Verification items for this drawing (mm, ordinates from the low corner). A direction names the side the tool comes from. Give positions to 0.01 mm unless a question says otherwise; leave off trailing zeros. Loops run counter-clockwise (first coordinate to the right, second up) from the corner with the lowest first, then second, coordinate; pieces in that order, holes last. Notation, with made-up numbers: M 24,62 L 69,62 A22 ccw 69,70 Z; hole C 87.5,-25.75 d3. An arc over 180 degrees is marked long. Answer in a Markdown table with one row per item.
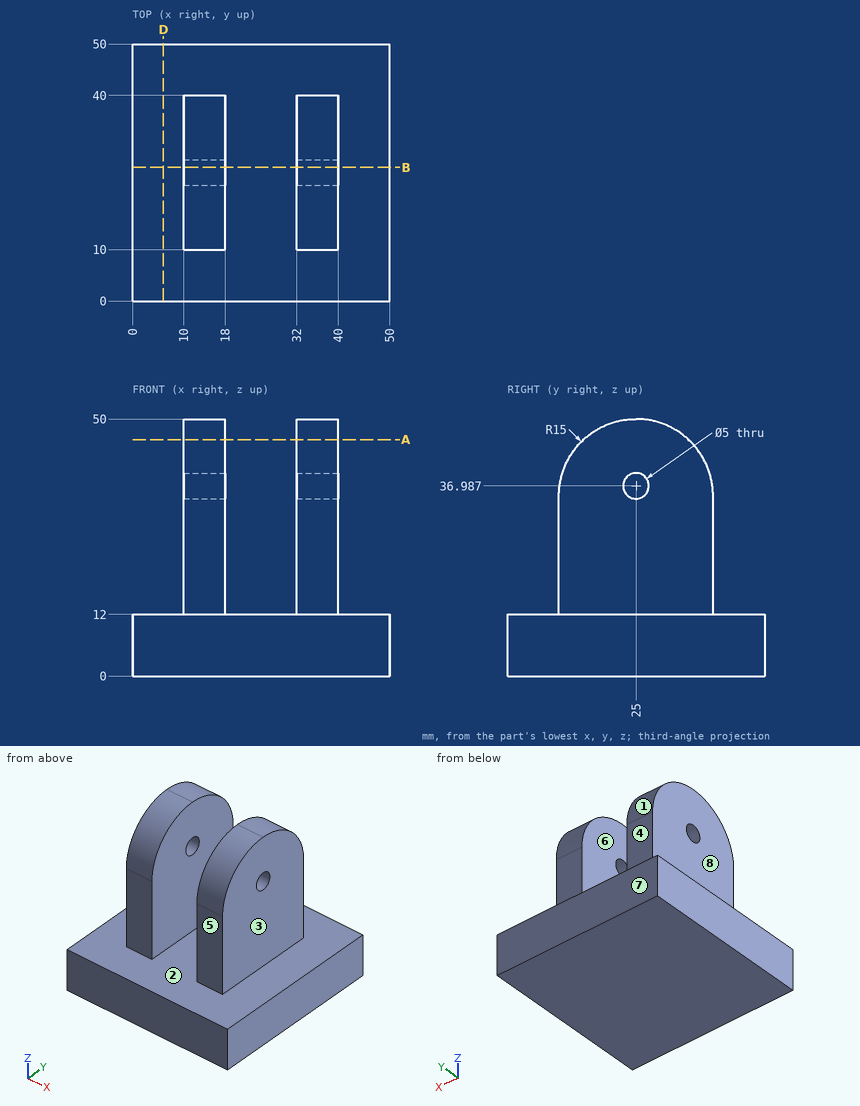
Item 1: Sectioned sample at B-B (y = 26). Record the cut outline in (x, z), and give its area (3 significant figures).
Reported:
| item | result |
|---|---|
| outline | M 0,0 L 50,0 L 50,12 L 40,12 L 40,34.7 L 32,34.7 L 32,12 L 18,12 L 18,34.7 L 10,34.7 L 10,12 L 0,12 Z; M 10,39.28 L 18,39.28 L 18,49.97 L 10,49.97 Z; M 32,39.28 L 40,39.28 L 40,49.97 L 32,49.97 Z |
| area | 1,130 mm^2 |
Item 2: Go/stop test with flat-tipped pins: pin 1 (8 mm diameter, centred on y = 43.5, z = 17, fed in from -X); pin 2 (4 mm diameter, centred on x = 35.5, z = 19.5, fed in from -Y); pin 3 (15 mm diameter, centred on y = 19, z = 39, fed in from +X). Record where each tip stops, or that it passes through.
Reported:
| item | result |
|---|---|
| pin 1 | stops at x = 10 |
| pin 2 | stops at y = 10 |
| pin 3 | stops at x = 40 |
Item 3: Scan lines: L1, parallel to X at y = 30.5, z = 21; L2, parallel to Z at x = 35, y = 25; L3, parallel to Y at x = 17.5, z = 15.5. Record each from-to range of solid material in increasing order. Write a range as [from, to].
Reported:
| item | result |
|---|---|
| L1 | x = [10, 18], [32, 40] |
| L2 | z = [0, 34.49], [39.49, 50] |
| L3 | y = [10, 40] |
Item 4: Tool access check on the marked faces 4, 5, 6, 7 and 8. Record the directions out of +Z, -Z, +X, -X, +Y, -Y that give a thin tool (end or side, any length) a straight path to the whole face; none if there is none.
Reported:
| item | result |
|---|---|
| face 4 | +Z, +X, -X, +Y |
| face 5 | +Z, +X, -X, -Y |
| face 6 | +Z, +Y, -Y |
| face 7 | +Z, -Z, +X, -X, +Y |
| face 8 | +Z, -X, +Y, -Y |
Item 5: Sectioned sample at A-A (z = 46). Record the cut outline in (x, y), and give its area (3 significant figures).
Reported:
| item | result |
|---|---|
| outline | M 10,14.8 L 18,14.8 L 18,35.2 L 10,35.2 Z; M 32,14.8 L 40,14.8 L 40,35.2 L 32,35.2 Z |
| area | 326 mm^2 |
Item 6: Sectioned sample at D-D (x = 6). Record the cut outline in (y, z), and give its area (3 significant figures).
Reported:
| item | result |
|---|---|
| outline | M 0,0 L 50,0 L 50,12 L 0,12 Z |
| area | 600 mm^2 |
Item 7: Release check for a two-part mould opening along X. For the marked faces 1, 2 and 3 record: released by +X, released by -X, zero draft, split by the parting line, or undercut.
Reported:
| item | result |
|---|---|
| face 1 | zero draft |
| face 2 | undercut |
| face 3 | released by +X |
